```python
from build123d import *

# Parameters (mm, degrees)
SKETCH_1_R      = 2
EXTRUDE_1_DEPTH = 5
FILLET_1_R      = 2.5
FILLET_2_R      = 2.5
FILLET_3_R      = 10


with BuildPart() as part:
    # 草圖1 → 填料-伸長1 (new body)
    with BuildSketch(Plane.XY):
        with BuildLine():
            Line((-17.000169764, -31.546546547), (-9.500169764, -6.546546547))
            Line((-9.500169764, -6.546546547), (-9.500169764, 96.553453453))
            Line((-9.500169764, 96.553453453), (-24.500169764, 96.553453453))
            Line((-24.500169764, 96.553453453), (-24.500169764, 86.553453453))
            ThreePointArc((-24.500169764, 86.553453453), (-28.500169764, 82.553453453), (-24.500169764, 78.553453453))
            Line((-24.500169764, 78.553453453), (-24.500169764, 52.453453453))
            ThreePointArc((-24.500169764, 52.453453453), (-28.500169764, 48.453453453), (-24.500169764, 44.453453453))
            Line((-24.500169764, 44.453453453), (-24.500169764, -31.546546547))
            Line((-24.500169764, -31.546546547), (-17.000169764, -31.546546547))
        make_face()
        with Locations((-24.500169764, 82.553453453)):
            Circle(SKETCH_1_R, mode=Mode.SUBTRACT)
        with Locations((-24.500169764, 48.453453453)):
            Circle(SKETCH_1_R, mode=Mode.SUBTRACT)
    extrude(amount=EXTRUDE_1_DEPTH)

    # 圓角1
    fillet_1_edges = [part.edges().sort_by_distance(p)[0] for p in [
        (-24.500169764, 96.553453453, 2.5),
        (-9.500169764, 96.553453453, 2.5),
        (-17.000169764, -31.546546547, 2.5),
        (-24.500169764, -31.546546547, 2.5),
    ]]
    fillet(fillet_1_edges, radius=FILLET_1_R)

    # 圓角2
    fillet_2_edges = [part.edges().sort_by_distance(p)[0] for p in [
        (-24.500169764, 44.453453453, 2.5),
        (-24.500169764, 52.453453453, 2.5),
        (-24.500169764, 78.553453453, 2.5),
    ]]
    fillet(fillet_2_edges, radius=FILLET_2_R)

    # 圓角3
    fillet_3_edges = [part.edges().sort_by_distance(p)[0] for p in [
        (-9.500169764, -6.546546547, 2.5),
    ]]
    fillet(fillet_3_edges, radius=FILLET_3_R)


solid = part.part
```
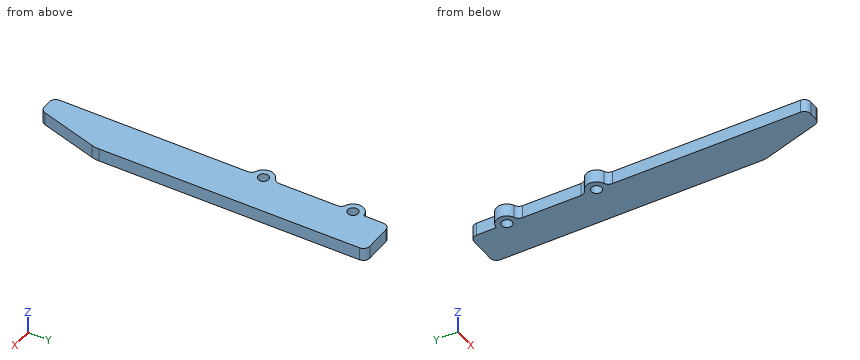
Design review of the part built by this model. Coordinates are the model's own, in mm. Give positions to 0.01 mm unless a question says otherwise; leave off trailing zeros. Write each loop counter-clockwise with the first axis right and the second up, starting at its lowest first coordinate (ties: lowest second). Pieces come first, ordered by that corner, then holes. Notation, with made-up numbers: (28.5, 5.25) - (44.5, 5.25) arc R25 ccw to (44.5, 19.25) - close; hole circle Ø7 at (24.25, 67.25). An arc over 180 degrees is marked (long way). Return JSON: item names as keys, results as strings. Group by question number.
(1) We need section C-C, the plane x = -15.25. Give the boundary of the cut face in (y, z), then the cut area to 3 significant figures.
(2) To check wall thickness, follow probe 1 along Y at (x, z) = (-26, 3.2); probe 2 along X at (y, z) = (25.5, 2); probe 3 along Y at (x, z) = (-18.75, 4.6). State the ranges of each line that lie inside material, in increasing order.
(3) We need section A-A, the plane z = 4.1. Give the boundary of the cut face in (x, y), then the cut area to 3 significant figures.
(4) Insertion check: pin 1 (2.5 mm diameter, centred on y = 0, z = 2, fed in from -X); pin 2 (8 mm diameter, centred on x = -16, y = 76, fed in from -Z); pin 3 (3 mm diameter, centred on x = -26.5, z = 3.5, fed in from -Y); pin 4 (2 mm diameter, centred on y = 54, z = 2.5, fed in from -X). Each pin has a flat end and moves straight along its axis. Give the tip position at first contact, or say it passes through.
(5) We need section B-B, the plane y = -4. Give the boundary of the cut face in (x, z).
Reported:
{
 "1": {"outline": "(-25.71, 0) - (96.55, 0) - (96.55, 5) - (-25.71, 5) - close", "area": "611 mm2"},
 "2": {"probe 1": "y = 44.74 to 47.13, 49.78 to 52.16, 78.84 to 81.23, 83.88 to 86.26", "probe 2": "x = -24.5 to -9.5", "probe 3": "y = -31.54 to 96.55"},
 "3": {"outline": "(-26.04, 44.76) arc R2.5 cw to (-24.5, 42.45) - (-24.5, -29.05) arc R2.5 ccw to (-22, -31.55) - (-18.86, -31.55) arc R2.5 ccw to (-16.47, -29.76) - (-9.92, -7.95) arc R10 ccw to (-9.5, -5.08) - (-9.5, 94.05) arc R2.5 ccw to (-12, 96.55) - (-22, 96.55) arc R2.5 ccw to (-24.5, 94.05) - (-24.5, 86.55) arc R4 ccw to (-26.04, 78.86) arc R2.5 cw to (-24.5, 76.55) - (-24.5, 54.45) arc R2.5 cw to (-26.04, 52.15) arc R4 ccw to start; hole circle Ø4 at (-24.5, 48.45); hole circle Ø4 at (-24.5, 82.55)", "area": "1,850 mm2"},
 "4": {"pin 1": "stops at x = -24.5", "pin 2": "stops at z = 0", "pin 3": "stops at y = 43.95", "pin 4": "stops at x = -24.97"},
 "5": {"outline": "(-24.5, 0) - (-9.5, 0) - (-9.5, 5) - (-24.5, 5) - close"}
}
